The model under review builds one solid part; all positions refer to its coordinate system, in mm. A direction names the side the tool comes from. Round coordinates to 2 decimals unless told otherwise and drop trailing zeros. Write each loop counter-clockwise with the first axis right and the second up, starting at its lowest first coordinate (ties: lowest second). Pieces come first, ordered by that corner, then holes.
Item 1: Draft analysis for pull direction X (two halves, no side actions). For faces 4 (the face through (48.521, 4.133, 1.095)), 5 (the face through (28.6, 7.7, 5.1)), 6 (the face through (0, 5, 5)), state which applies: +X half, -X half, draft (parallel to the pull), parting line (faces both ways), or undercut.
Item 2: Add section D-D (x = 5). Give the boundary of the cut face in (y, z), plus the area to 3 significant figures.
Item 3: Add section A-A (y = 5). Give the boundary of the cut face in (x, z).
Item 4: Add section C-C (x = 32). Give the boundary of the cut face in (y, z).
Item 5: Machinability: for faces 1 (the face through (47, 5, 5)), 2 (the face through (25, 10, 5)), 3 (the face through (-1.48, 5.98, 9.39)), which of the approach directions +Z, -Z, +X, -X, +Y, -Y give a long, thin tool a straight path to every point of the face, cutting with its end or side? Answer none if there is none.
Item 6: To check wall thickness, follow L1, parallel to Z at x = 48.4, y = 5; L2, parallel to X at y = 6.5, z = 8.5; L3, parallel to Y at x = 5, z = 6. State the ranges of each line that lie inside material, in increasing order.
Item 7: Clearance check with a flat-ended pin moving along its axis: pin 1 Ø2.5 at (y, z) = (5.5, 3) entering from +X. State where the tip first meets the part, or that it passes through.
Item 8: Add section B-B (z = 5). Give the boundary of the cut face in (x, y), plus the area to 3 significant figures.
Autodesk Fusion 360 part; units mm, degrees
sketch "Sketch1" plane through (0, 0, 0) normal (0, 0, 1) x (1, 0, 0)
  line L0 (0, 0) -> (50, 0)
  line L1 (50, 0) -> (50, 10)
  line L2 (50, 10) -> (0, 10)
  line L3 (0, 10) -> (0, 0)
  dimension "d1" = 50
  dimension "d2" = 10
extrude "Extrude1" add sketch "Sketch1" along normal blind 10
sketch "Sketch2" plane through (0, 0, 10) normal (0, 0, 1) x (-1, 0, 0)
  line L0 (0, -10) -> (0, 0)
  line L1 (0, 0) -> (-50, 0)
  line L2 (-50, 0) -> (-50, -10)
  line L3 (-50, -10) -> (0, -10)
  circle A0 centre (-5, -5) radius 4.5
  circle A1 centre (-25, -5) radius 4.5
  dimension "d5" = 9
  dimension "d6" = 9
extrude "Extrude2" cut sketch "Sketch2" against normal blind 11 contours A0 | A1
sketch "Sketch3" plane through (50, 0, 0) normal (1, 0, 0) x (0, 1, 0)
  line L0 (0, 0) -> (10, 0)
  line L1 (10, 0) -> (10, 10)
  line L2 (10, 10) -> (0, 10)
  line L3 (0, 10) -> (0, 0)
  circle A0 centre (5, 5) radius 4
  dimension "d9" = 8
extrude "Extrude3" cut sketch "Sketch3" against normal blind 3 contours A0
sketch "Sketch4" plane through (0, 0, 0) normal (0, -1, 0) x (1, 0, 0)
  line L0 (0, 0) -> (50, 0)
  line L1 (50, 0) -> (50, 10)
  line L2 (50, 10) -> (0, 10)
  line L3 (0, 10) -> (0, 0)
  circle A0 centre (15, 5) radius 4.5
  circle A1 centre (35, 5) radius 4.5
  dimension "d12" = 9
  dimension "d13" = 9
extrude "Extrude4" cut sketch "Sketch4" against normal blind 20 contours A0 | A1
sketch "Sketch5" plane through (0, 0, 0) normal (-1, 0, 0) x (0, -1, 0)
  line L0 (-10, 0) -> (0, 0)
  line L1 (0, 0) -> (0, 10)
  line L2 (0, 10) -> (-10, 10)
  line L3 (-10, 10) -> (-10, 0)
  circle A0 centre (-5, 5) radius 4.5
  circle A1 centre (-5, 5) radius 4
  dimension "d16" = 9
  dimension "d17" = 8
extrude "Extrude5" add sketch "Sketch5" along normal blind 3 contours A0
Numbers:
1. face 4: draft
1. face 5: undercut
1. face 6: -X half
2. outline: (0, 0) - (0.5, 0) - (0.5, 10) - (0, 10) - close; (9.5, 0) - (10, 0) - (10, 10) - (9.5, 10) - close
2. area: 10.0 mm2
3. outline: (-3, 0.5) - (0, 0.5) - (0, 0) - (0.5, 0) - (0.5, 10) - (0, 10) - (0, 9.5) - (-3, 9.5) - (-3, 9) - (0, 9) - (0, 1) - (-3, 1) - close; (9.5, 0) - (20.5, 0) - (20.5, 10) - (9.5, 10) - close; (29.5, 0) - (50, 0) - (50, 1) - (47, 1) - (47, 9) - (50, 9) - (50, 10) - (29.5, 10) - close; hole circle Ø9 at (15, 5); hole circle Ø9 at (35, 5)
4. outline: (0, 0) - (10, 0) - (10, 1.65) - (0, 1.65) - close; (0, 8.35) - (10, 8.35) - (10, 10) - (0, 10) - close
5. face 1: +X
5. face 2: +Z, -Z, +X, -X, +Y
5. face 3: -X
6. L1: z = 0 to 1, 9 to 10
6. L2: x = 0 to 0.76, 9.24 to 12.17, 17.83 to 20.76, 29.24 to 32.17, 37.83 to 47
6. L3: y = 0 to 0.5, 9.5 to 10
7. pin 1: stops at x = 47
8. outline: (-3, 0.5) - (0, 0.5) - (0, 0) - (10.5, 0) - (10.5, 10) - (0, 10) - (0, 9.5) - (-3, 9.5) - (-3, 9) - (0, 9) - (0, 1) - (-3, 1) - close; (19.5, 0) - (30.5, 0) - (30.5, 10) - (19.5, 10) - close; (39.5, 0) - (50, 0) - (50, 1) - (47, 1) - (47, 9) - (50, 9) - (50, 10) - (39.5, 10) - close; hole circle Ø9 at (5, 5); hole circle Ø9 at (25, 5)
8. area: 172 mm2
